```python
from build123d import *

# Parameters (mm, degrees)
F0_W     = 152.4
F0_H     = 100.554315
F0_R     = 23.747054
F1_DEPTH = 12.7


with BuildPart() as f1:
    # F0 (on Top) → F1 (new body)
    with BuildSketch(Plane.XY):
        with Locations((0.451705, 0.590802)):
            Rectangle(F0_W, F0_H)
        with BuildLine():
            ThreePointArc((-57.500403, 29.078691), (-62.083381, 40.142978), (-51.019094, 35.56))
            Line((-51.019094, 35.56), (50.968102, 35.56))
            ThreePointArc((50.968102, 35.56), (57.500403, 42.092301), (64.032704, 35.56))
            ThreePointArc((64.032704, 35.56), (62.119438, 30.940966), (57.500403, 29.027699))
            Line((57.500403, 29.027699), (57.500403, -29.139609))
            ThreePointArc((57.500403, -29.139609), (62.040305, -31.020098), (63.920794, -35.56))
            ThreePointArc((63.920794, -35.56), (57.500403, -41.980391), (51.080013, -35.56))
            Line((51.080013, -35.56), (-51.003335, -35.56))
            ThreePointArc((-51.003335, -35.56), (-62.094525, -40.154121), (-57.500403, -29.062932))
            Line((-57.500403, -29.062932), (-57.500403, 29.078691))
        make_face(mode=Mode.SUBTRACT)
        with BuildLine():
            Line((50.968102, 35.56), (-51.019094, 35.56))
            ThreePointArc((-51.019094, 35.56), (-52.917426, 30.977022), (-57.500403, 29.078691))
            Line((-57.500403, 29.078691), (-57.500403, -29.062932))
            ThreePointArc((-57.500403, -29.062932), (-52.906282, -30.965879), (-51.003335, -35.56))
            Line((-51.003335, -35.56), (51.080013, -35.56))
            ThreePointArc((51.080013, -35.56), (52.960502, -31.020098), (57.500403, -29.139609))
            Line((57.500403, -29.139609), (57.500403, 29.027699))
            ThreePointArc((57.500403, 29.027699), (52.881369, 30.940966), (50.968102, 35.56))
        make_face()
        with Locations((0.451705, 0.590802)):
            Circle(F0_R, mode=Mode.SUBTRACT)
    extrude(amount=F1_DEPTH)


solid = f1.part
```
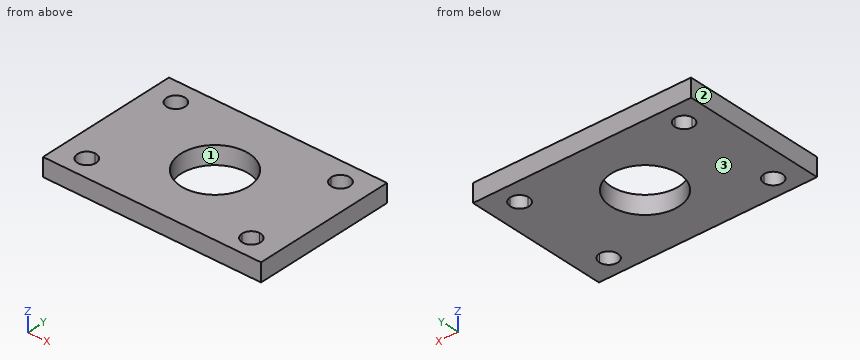
Could you check a few things on this model? Use its own coordinates, in mm. Face numbers are marked on the shaded views. Coordinates: 2 decimals unless noted, no trailing zeros. Write each loop counter-clockwise with the first axis right and the second up, starting at its lowest first coordinate (ties: lowest second). Pieces come first, ordered by that corner, then holes. Notation, with made-up numbers: (69.25, 87) -> (97.25, 87) arc R26 cw to (97.25, 104) -> close; hole circle Ø10 at (-25, 23). An arc over 180 degrees is marked (long way). One line per question, with ' | ' between items. Start each with the question number.
1. If we section it at D-D (z = 2.5): Please give me the cut outline in (x, y).
2. If we section it at B-B (x = -7.5): Please give me the cut outline in (y, z), and give its area (3 significant figures).
3. Please list where these lines run through material, in increasing order: line 1 along X through (y, z) = (-35.56, 6); line 2 along X through (y, z) = (35.56, 4.5); line 3 along Y through (x, z) = (55, 4).
4. Will this pin go through, and if not, where does the flat tip stop? P1, Ø15, axis at x = -57.5, y = -35.56, coming from the +Z side.
5. Thinking about a two-plate mould opening in X: for the marked faces 1, 2 and 3, which applies, pulls with the +X half, pulls with the -X half, needs draft (parallel to the pull), parting line crosses it, or undercut?
6. If we section it at C-C (y = 38.5): Please give me the cut outline in (x, z), and give its area (3 significant figures).
7. If we section it at A-A (y = -7.5): Please give me the cut outline in (x, z).
Return value:
1) outline: (-75.75, -49.69) -> (76.65, -49.69) -> (76.65, 50.87) -> (-75.75, 50.87) -> close; hole circle Ø12.99 at (-57.5, -35.56); hole circle Ø12.96 at (-57.5, 35.56); hole circle Ø47.49 at (0.45, 0.59); hole (50.97, 35.56) arc R6.53 ccw to (57.5, 29.03) arc R6.53 ccw (long way) to start; hole (51.08, -35.56) arc R6.42 ccw (long way) to (57.5, -29.14) arc R6.42 ccw to start
2) outline: (-49.69, 0) -> (-21.79, 0) -> (-21.79, 12.7) -> (-49.69, 12.7) -> close; (22.97, 0) -> (50.87, 0) -> (50.87, 12.7) -> (22.97, 12.7) -> close | area: 709 mm²
3) line 1: x = -75.75 to -64, -51 to 51.08, 63.92 to 76.65 | line 2: x = -75.75 to -63.98, -51.02 to 50.97, 64.03 to 76.65 | line 3: y = -49.69 to -41.47, -29.65 to 29.53, 41.59 to 50.87
4) P1: stops at z = 12.7
5) face 1: undercut | face 2: pulls with the -X half | face 3: needs draft
6) outline: (-75.75, 0) -> (-63.28, 0) -> (-63.28, 12.7) -> (-75.75, 12.7) -> close; (-51.72, 0) -> (51.67, 0) -> (51.67, 12.7) -> (-51.72, 12.7) -> close; (63.33, 0) -> (76.65, 0) -> (76.65, 12.7) -> (63.33, 12.7) -> close | area: 1,640 mm²
7) outline: (-75.75, 0) -> (-21.87, 0) -> (-21.87, 12.7) -> (-75.75, 12.7) -> close; (22.78, 0) -> (76.65, 0) -> (76.65, 12.7) -> (22.78, 12.7) -> close
